Part model, mm, in its own coordinate system. Face numbers are marked on the shaded views. A direction names the side the tool comes from. Round coordinates to 2 decimals unless told otherwise and drop trailing zeros. Loops run counter-clockwise (first coordinate to the right, second up) from the corner with the lowest first, then second, coordinate; pieces in that order, holes last. Notation, with made-up numbers: M 35.25,-31.75 L 51.25,-31.75 A10 cw 51.25,-16.75 Z; hole C -13.5,63.5 d2. An arc over 180 degrees is marked long. Answer as CSV lines item,"result". Start each with the question number.
Item 1: Band-saw the part on B-B (z = 5.75). Give the cut face in (x, y), and give its area (3 significant figures).
Item 2: Drop flat-ended pins along their axis: pin 1 Ø6 at (x, y) = (3.5, 0) entering from +Z; pin 2 Ø3 at (x, z) = (9.5, 5.75) entering from -Y; pin 3 Ø3 at (x, y) = (-9, 0) entering from +Z. Give the stop position or say it passes through.
Item 3: Which spindle directions (+Z, -Z, +X, -X, +Y, -Y) get a long thin tool onto all of the face, cutting with end or side? Do the marked faces 1 and 2. Say none if no direction does.
Item 4: Band-saw the part on A-A (x = 3.5). Give the cut face in (y, z), and give its area (3 significant figures).
Item 5: Wall check: line 1 (X direction, y = 0, z = 7.75); line 2 (X direction, y = -0.5, z = 8); line 3 (Z direction, x = 9.5, y = 4). Give the ranges that are in metal, low to high.
Item 6: Band-saw the part on D-D (x = -9). Give the cut face in (y, z).
Item 7: Band-saw the part on C-C (y = 4.75). Give the cut face in (x, z), and give its area (3 significant figures).
Item 8: Mould opens along X. For the marked faces 3, 4, 5 and 6 say: pulls with the +X half, pulls with the -X half, needs draft (parallel to the pull), parting line crosses it, or undercut.
```python
from build123d import *

# Parameters (mm, degrees)
F0_W           = 23
F0_H           = 16
F1_DEPTH       = 11.5
F3_D           = 5
F3_CSINK_D     = 6.5
F3_CSINK_ANGLE = 90
F4_D           = 2.5
F4_CSINK_D     = 3.2
F4_CSINK_ANGLE = 90
F5_R           = 1.55
F6_DEPTH       = 16.001
F8_D           = 2.5
F8_DEPTH       = 5.75
F8_CSINK_D     = 3.2
F8_CSINK_ANGLE = 90
F8_TIP         = 0.7510757738


with BuildPart() as f1:
    # F0 (on Top) → F1 (new body)
    with BuildSketch(Plane.XY):
        Rectangle(F0_W, F0_H)
    extrude(amount=F1_DEPTH)

    # F3 (through all)
    with Locations(Plane.XY.offset(11.5)):
        with Locations((3.5, 0)):
            CounterSinkHole(F3_D / 2, F3_CSINK_D / 2, counter_sink_angle=F3_CSINK_ANGLE)

    # F4 (through all)
    with Locations(Plane.XY.offset(11.5)):
        with Locations((-9, 0)):
            CounterSinkHole(F4_D / 2, F4_CSINK_D / 2, counter_sink_angle=F4_CSINK_ANGLE)

    # F5 (on face) → F6 (cut, through all)
    with BuildSketch(Plane.XZ.offset(8)):
        with BuildLine():
            Line((-4.589129705, 5), (-5.8284271247, 5))
            ThreePointArc((-5.8284271247, 5), (-6, 4), (-5.8284271247, 3))
            Line((-5.8284271247, 3), (-4.589129705, 3))
            Line((-4.589129705, 3), (-4.589129705, 5))
        make_face()
        with BuildLine():
            ThreePointArc((-5.8284271247, 3), (-2.4926940638, 1.043204321), (0, 4))
            ThreePointArc((0, 4), (-2.4926940638, 6.956795679), (-5.8284271247, 5))
            Line((-5.8284271247, 5), (-4.589129705, 5))
            Line((-4.589129705, 5), (-4.589129705, 3))
            Line((-4.589129705, 3), (-5.8284271247, 3))
        make_face()
        with Locations((9.5, 5.75)):
            Circle(F5_R)
        with BuildLine():
            ThreePointArc((-5.8284271247, 3), (-6, 4), (-5.8284271247, 5))
            Line((-5.8284271247, 5), (-11.5, 5))
            Line((-11.5, 5), (-11.5, 3))
            Line((-11.5, 3), (-5.8284271247, 3))
        make_face()
    extrude(amount=-F6_DEPTH, mode=Mode.SUBTRACT)

    # F8
    with Locations(Plane(origin=(0, 0, 0), x_dir=(1, 0, 0), z_dir=(0, 0, -1))):
        with Locations((9.7161801532, 0)):
            CounterSinkHole(F8_D / 2, F8_CSINK_D / 2, depth=F8_DEPTH, counter_sink_angle=F8_CSINK_ANGLE)
            with Locations((0, 0, -(F8_DEPTH + F8_TIP / 2))):  # 118° drill point
                Cone(0, F8_D / 2, F8_TIP, mode=Mode.SUBTRACT)


solid = f1.part
```
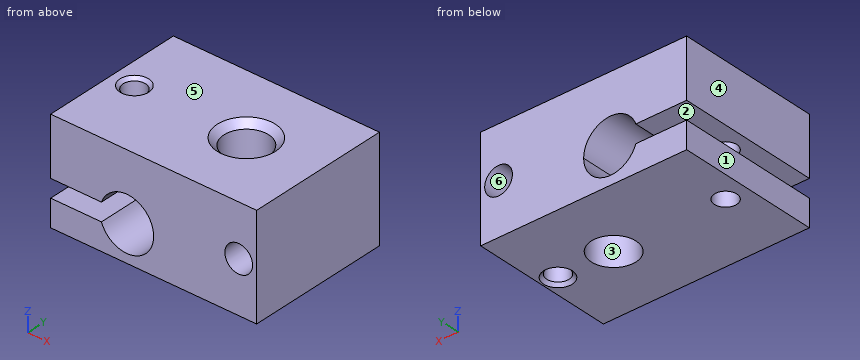
Answer block:
1,outline,"M -11.5,-8 L -5.44,-8 L -5.44,8 L -11.5,8 Z; M -0.56,-8 L 7.95,-8 L 7.95,8 L -0.56,8 Z; M 11.05,-8 L 11.5,-8 L 11.5,8 L 11.05,8 Z; hole C -9,0 d2.5; hole C 3.5,0 d5"
1,area,"216 mm^2"
2,pin 1,"stops at z = 11.25"
2,pin 2,"passes through"
2,pin 3,"stops at z = 11.4"
3,face 1,"+Z, -Z, -X, +Y, -Y"
3,face 2,"-X, +Y, -Y"
4,outline,"M -8,0 L -2.5,0 L -2.5,10.75 L -3.25,11.5 L -8,11.5 Z; M 2.5,0 L 8,0 L 8,11.5 L 3.25,11.5 L 2.5,10.75 Z"
4,area,"126 mm^2"
5,line 1,"x = -11.5 to -10.25, -7.75 to 1, 6 to 11.5"
5,line 2,"x = -11.5 to -10.15, -7.85 to 1.05, 5.95 to 11.5"
5,line 3,"z = 0 to 4.2, 7.3 to 11.5"
6,outline,"M -8,0 L -1.25,0 L -1.25,3 L -8,3 Z; M -8,5 L -1.25,5 L -1.25,11.15 L -1.6,11.5 L -8,11.5 Z; M 1.25,0 L 8,0 L 8,3 L 1.25,3 Z; M 1.25,5 L 8,5 L 8,11.5 L 1.6,11.5 L 1.25,11.15 Z"
7,outline,"M -11.5,0 L 11.5,0 L 11.5,11.5 L -11.5,11.5 L -11.5,5 L -5.83,5 A3 cw long -5.83,3 L -11.5,3 Z; hole C 9.5,5.75 d3.1"
7,area,"218 mm^2"
8,face 3,"undercut"
8,face 4,"pulls with the -X half"
8,face 5,"needs draft"
8,face 6,"undercut"
